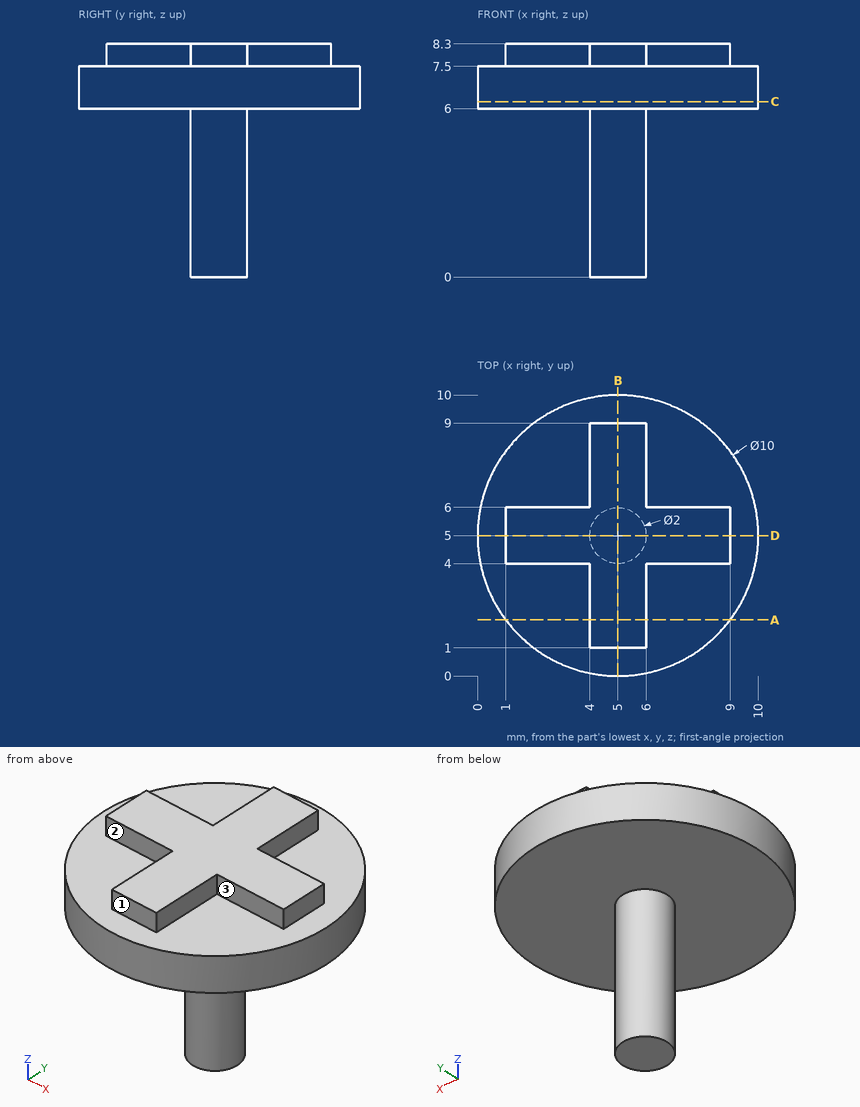
Could you check a few things on this drawing? It's one solid part, dimensions in mm from its lowest x, y, z. A direction names the side the tool comes from. Give positions to 0.01 mm unless a question says otherwise; leave off trailing zeros. Order: outer loops, then holes, each group sorted by start corner. A loop starts at its lowest first (then second) coordinate and runs counter-clockwise, first axis right, second up. Notation, with made-up numbers: M 45.5,-34.5 L 103.5,-34.5 A19 ccw 103.5,-9.5 Z; hole C 5,75 d8. An arc over 180 degrees is marked long. Use one line per item in the form item = value.
Item 1: For the marked faces 1, 2 and 3, which set-ups out of +Z, -Z, +X, -X, +Y, -Y let a thin tool reach every point of the face, with its end or its side?
Values follow:
face_1 = +Z, +X, -X, -Y
face_2 = +Z, -X, -Y
face_3 = +Z, +X, -Y
Item 2: If we section it at A-A, the plane y = 2: Write out the boundary of the cut face in (x, z), and give its area (3 significant figures).
Values follow:
outline = M 1,6 L 9,6 L 9,7.5 L 6,7.5 L 6,8.3 L 4,8.3 L 4,7.5 L 1,7.5 Z
area = 13.6 mm^2
Item 3: If we section it at C-C, the plane z = 6.25: Write out the boundary of the cut face in (x, y), and give its area (3 significant figures).
Values follow:
outline = C 5,5 d10
area = 78.5 mm^2
Item 4: Will these pins go through, and if not, where does the flat tip stop? pin 1 Ø0.9 at (y, z) = (5, 8) entering from -X; pin 2 Ø0.6 at (y, z) = (3, 8) entering from -X; pin 3 Ø0.9 at (x, z) = (2.5, 8) entering from +Y.
Values follow:
pin_1 = 1
pin_2 = 4
pin_3 = 6
Item 5: If we section it at B-B, the plane x = 5: Write out the boundary of the cut face in (y, z), and give its area (3 significant figures).
Values follow:
outline = M 0,6 L 4,6 L 4,0 L 6,0 L 6,6 L 10,6 L 10,7.5 L 9,7.5 L 9,8.3 L 1,8.3 L 1,7.5 L 0,7.5 Z
area = 33.4 mm^2
Item 6: If I drill on line 1 along Z through (x, y) = (8, 8.25); line 2 along Z through (x, y) = (5.5, 7.25); line 3 along Y through (x, z) = (3.5, 7.75), over which ranges is the centre line in solid material (lowest first)? Write a range as [from, to].
Values follow:
line_1 = [6, 7.5]
line_2 = [6, 8.3]
line_3 = [4, 6]
